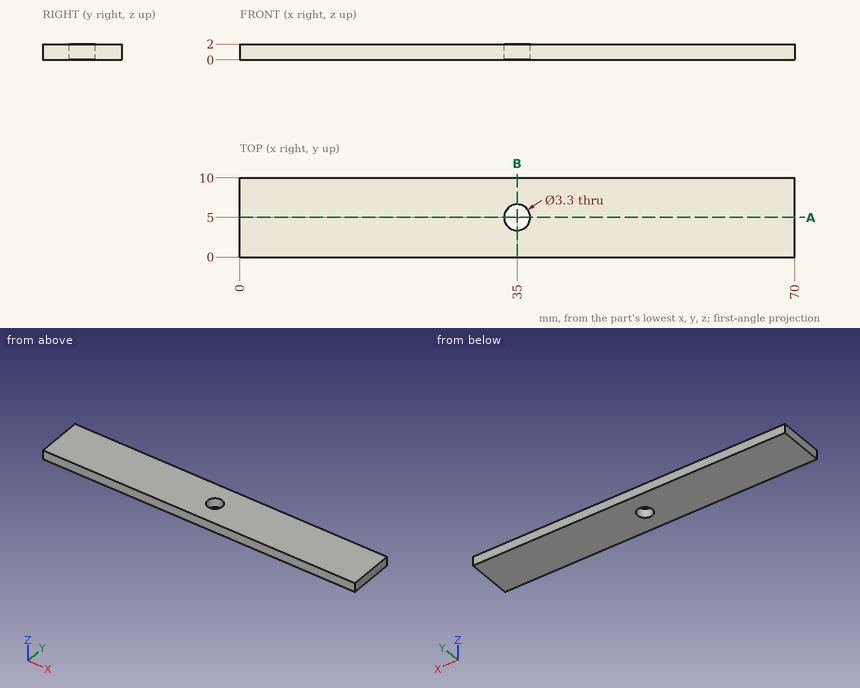
Study the drawing (mm; zero at the part's minimum x, y, z) and answer. Coordinates: 2 decimals unless noted, no trailing zeros. Loops run counter-clockwise (first coordinate to the right, second up) from the corner with the lowest first, then second, coordinate; pieces in that order, holes last. Notation, with made-up numbers: (-26.5, 74) -> (17.5, 74) arc R37 ccw to (17.5, 112) -> close; hole circle Ø8 at (62.5, 34.5). An arc over 180 degrees is marked (long way). Answer as CSV lines item,"result".
1) Straight lines are drawn through the part: probe 1 along Y at (x, z) = (35, 1.3); probe 2 along X at (y, z) = (4, 1.2). For each, find the intervals that lie inside material, in ascending order.
A:
probe 1,"y = 0 to 3.35, 6.65 to 10"
probe 2,"x = 0 to 33.69, 36.31 to 70"
2) A flat-ended cylindrical pin translates along its axis: pin 1 (2 mm diameter, centred on x = 35, y = 5, fed in from -Z). Find the tip coordinate at first contact, or state that the pin passes through.
A:
pin 1,"passes through"
3) The part is cut by section A-A (y = 5). Give the vertices of the cut face in (x, z), and give its area (3 significant figures).
A:
outline,"(0, 0) -> (33.35, 0) -> (33.35, 2) -> (0, 2) -> close; (36.65, 0) -> (70, 0) -> (70, 2) -> (36.65, 2) -> close"
area,"133 mm²"
4) The part is cut by section B-B (x = 35). Give the vertices of the cut face in (y, z), and give its area (3 significant figures).
A:
outline,"(0, 0) -> (3.35, 0) -> (3.35, 2) -> (0, 2) -> close; (6.65, 0) -> (10, 0) -> (10, 2) -> (6.65, 2) -> close"
area,"13.4 mm²"
